Read the model definition and answer for the solid it produces. Units are mm, in the model's axes. Face numbers are marked on the shaded views. A direction names the side the tool comes from. Give positions to 0.01 mm unless a question says otherwise; leave off trailing zeros. Order: outer loops, then holes, each group sorted by start corner. A loop starts at its lowest first (then second) coordinate and runs counter-clockwise, first axis right, second up. Notation, with made-up numbers: (60, 42.25) - (82, 42.25) arc R13 cw to (82, 52.25) - close; hole circle Ø5 at (30.25, 54). An arc over 180 degrees is marked (long way). One line per item, written item: value. Start each with the question number.
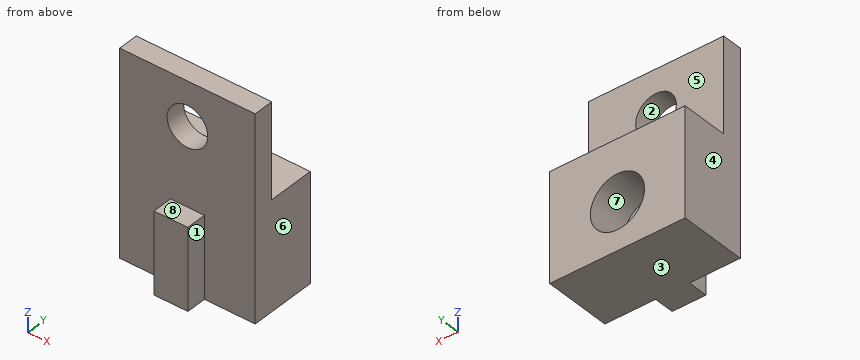
```python
from build123d import *

# Parameters (mm, degrees)
SKETCH1_W               = 20
SKETCH1_H               = 30
BOSS_EXTRUDE1_DEPTH     = 3
SKETCH2_W               = 5
SKETCH2_H               = 12
BOSS_EXTRUDE2_DEPTH     = 3
SKETCH3_R               = 7
SKETCH3_R_2             = 4
BOSS_EXTRUDE3_DEPTH     = 7
SKETCH4_R               = 4
BOSS_EXTRUDE4_DEPTH     = 1
CUT_EXTRUDE1_DEPTH      = 20.339079606
CUT_EXTRUDE1_DEPTH_BACK = 20.339079606
SKETCH5_R               = 3
SKETCH6_R               = 7
SKETCH6_R_2             = 4
BOSS_EXTRUDE6_DEPTH     = 7


with BuildPart() as part:
    # Sketch1 → Boss-Extrude1 (new body)
    with BuildSketch(Plane(origin=(0, 0, 0), x_dir=(1, 0, 0), z_dir=(0, 1, 0))):
        Rectangle(SKETCH1_W, SKETCH1_H)
    extrude(amount=BOSS_EXTRUDE1_DEPTH)

    # Sketch2 → Boss-Extrude2 (add)
    with BuildSketch(Plane.XZ):
        with Locations((0, -9)):
            Rectangle(SKETCH2_W, SKETCH2_H)
    extrude(amount=BOSS_EXTRUDE2_DEPTH)

    # Sketch3 → Boss-Extrude3 (add)
    with BuildSketch(Plane(origin=(0, 3, 0), x_dir=(1, 0, 0), z_dir=(0, 1, 0))):
        with Locations(Location((0, 8, 0), (0, 0, 90))):
            Circle(SKETCH3_R)
        with Locations(Location((0, 8, 0), (0, 0, 270))):
            Circle(SKETCH3_R_2, mode=Mode.SUBTRACT)
    extrude(amount=BOSS_EXTRUDE3_DEPTH)

    # Sketch4 → Boss-Extrude4 (add)
    with BuildSketch(Plane(origin=(0, 3, 0), x_dir=(1, 0, 0), z_dir=(0, 1, 0))):
        with Locations(Location((0, 8, 0), (0, 0, 270))):
            Circle(SKETCH4_R)
    extrude(amount=BOSS_EXTRUDE4_DEPTH)

    # Sketch5 → Cut-Extrude1 (cut, two sides: drawn at the far end of the back side and taken through both)
    with BuildSketch(Plane(origin=(0, 3, 0), x_dir=(1, 0, 0), z_dir=(0, 1, 0)).offset(-CUT_EXTRUDE1_DEPTH_BACK)):
        with Locations(Location((0, -8.5, 0), (0, 0, 90))):
            Circle(SKETCH5_R)
    extrude(amount=CUT_EXTRUDE1_DEPTH + CUT_EXTRUDE1_DEPTH_BACK, mode=Mode.SUBTRACT)

    # Sketch6 → Boss-Extrude6 (add)
    # profile 1 of 2: a face of its own
    with BuildSketch(Plane(origin=(0, 3, 0), x_dir=(1, 0, 0), z_dir=(0, 1, 0))):
        Polygon((0, 15), (-10, 15), (-10, -1), (10, -1), (10, 15), align=None)
        with BuildLine():
            ThreePointArc((7, 8), (-4.949747468, 3.050252532), (0, 15))
            ThreePointArc((0, 15), (4.949747468, 12.949747468), (7, 8))
        make_face(mode=Mode.SUBTRACT)
    # profile 2 of 2: a face of its own
    with BuildSketch(Plane(origin=(0, 3, 0), x_dir=(1, 0, 0), z_dir=(0, 1, 0))):
        with Locations((0, 8)):
            Circle(SKETCH6_R)
        with Locations(Location((0, 8, 0), (0, 0, 270))):
            Circle(SKETCH6_R_2, mode=Mode.SUBTRACT)
    extrude(amount=BOSS_EXTRUDE6_DEPTH)


solid = part.part
```
1) Each of these flat-tipped pins is pushed along its axis until it touches: pin 1 (1.5 mm diameter, centred on x = 6.5, y = -1, fed in from +Z); pin 2 (6 mm diameter, centred on x = 5, y = 8, fed in from +Z); pin 3 (11 mm diameter, centred on x = 0.5, z = 8, fed in from +Y); pin 4 (10 mm diameter, centred on x = 8, z = 11, fed in from -Y). Where does it stop, or does it pass through?
2) The mould has two halves that part along Z. Classify the marked faces 1, 2 and 3: +Z half, -Z half, draft (parallel to the pull), parting line (faces both ways), or undercut.
3) Section B-B on x = 0 is taken. Write down the section's boundary in (y, z).
4) Section A-A on z = 8.5 is taken. Write down the section's boundary in (x, y).
5) Section D-D on x = -6 is taken. Write down the section's boundary in (y, z), plus the area to 3 significant figures.
6) Find the intervals of material crossed by probe 1 along X at (y, z) = (2.35, 8.5); probe 2 along X at (y, z) = (8.7, -8); probe 3 along Y at (x, z) = (-6, -5), in increasing order. Write a range as from..to.
7) Section C-C on y = 0.5 is taken. Write down the section's boundary in (x, z).
8) For the marked faces 4, 5, 6, 7 and 8, determine the directions among +Z, -Z, +X, -X, +Y, -Y from which every point of the face is accessible in a straight line to the end or side of a thin tool.
Solved:
1. pin 1: passes through
1. pin 2: stops at z = 1
1. pin 3: stops at y = 3
1. pin 4: stops at y = 0
2. face 1: draft
2. face 2: undercut
2. face 3: -Z half
3. outline: (-3, -15) - (10, -15) - (10, -12) - (4, -12) - (4, -4) - (10, -4) - (10, 1) - (3, 1) - (3, 5.5) - (0, 5.5) - (0, -3) - (-3, -3) - close; (0, 11.5) - (3, 11.5) - (3, 15) - (0, 15) - close
4. outline: (-10, 0) - (-3, 0) - (-3, 3) - (-10, 3) - close; (3, 0) - (10, 0) - (10, 3) - (3, 3) - close
5. outline: (0, -15) - (10, -15) - (10, 1) - (3, 1) - (3, 15) - (0, 15) - close
5. area: 202 mm2
6. probe 1: x = -10..-3, 3..10
6. probe 2: x = -10..-4, 4..10
6. probe 3: y = 0..10
7. outline: (-10, -15) - (10, -15) - (10, 15) - (-10, 15) - close; hole circle Ø6 at (0, 8.5)
8. face 4: +Z, -Z, -X, +Y, -Y
8. face 5: +Z, +X, -X, +Y
8. face 6: +Z, -Z, +X, +Y, -Y
8. face 7: +Y
8. face 8: +Z, +X, -X, -Y
